Model file for the job. Use its own axes, mm. Face numbers are marked on the shaded views. A direction names the side the tool comes from. Coordinates: 2 decimals unless noted, no trailing zeros. Write each loop counter-clockwise with the first axis right and the second up, starting at its lowest first coordinate (ties: lowest second). Pieces come first, ordered by that corner, then holes. Notation, with made-up numbers: M 73.5,85 L 88.5,85 A14 cw 88.5,91 Z; hole C 3.5,-4 d2. An arc over 180 degrees is marked long. Answer in a Markdown table with one row per item. Add a question column.
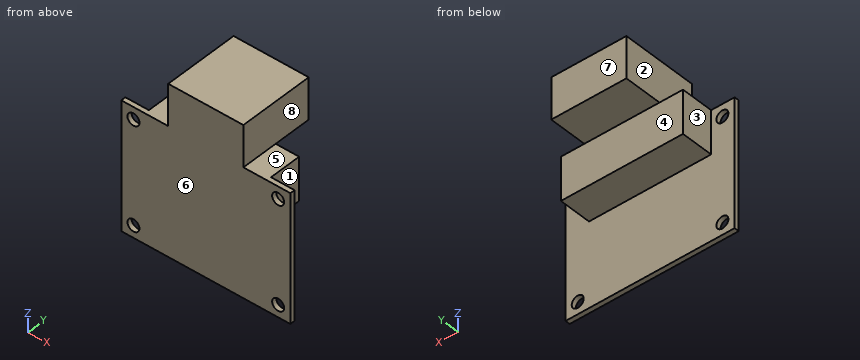
```python
from build123d import *

# Parameters (mm, degrees)
SKETCH1_W            = 45
SKETCH1_H            = 45
BOSS_EXTRUDE1_DEPTH  = 10.033
SKETCH2_W            = 12.5
SKETCH2_H            = 11
CUT_EXTRUDE1_DEPTH   = 20.066
CUT_EXTRUDE2_DEPTH   = 18.796
CUT_EXTRUDE3_DEPTH   = 10.16
M3_CLEARANCE_HOLE1_D = 3.2


with BuildPart() as part:
    # Sketch1 → Boss-Extrude1 (new, symmetric)
    with BuildSketch(Plane(origin=(0, 0, 0), x_dir=(1, 0, 0), z_dir=(0, 1, 0))):
        Rectangle(SKETCH1_W, SKETCH1_H)
    extrude(amount=BOSS_EXTRUDE1_DEPTH, both=True)

    # Sketch2 → Cut-Extrude1 (cut)
    with BuildSketch(Plane(origin=(0, 10.033, 0), x_dir=(1, 0, 0), z_dir=(0, 1, 0))):
        with Locations((16.25, -17)):
            Rectangle(SKETCH2_W, SKETCH2_H)
    cut_extrude1 = extrude(amount=-CUT_EXTRUDE1_DEPTH, mode=Mode.SUBTRACT)

    # Mirror1: Cut-Extrude1 across plane
    add(cut_extrude1.mirror(Plane(origin=(0, 0, 0), x_dir=(0, 0, 1), z_dir=(1, 0, 0))), mode=Mode.SUBTRACT)

    # Sketch3 → Cut-Extrude2 (cut)
    with BuildSketch(Plane(origin=(0, 10.033, 0), x_dir=(1, 0, 0), z_dir=(0, 1, 0))):
        Polygon((-22.5, -11.5), (-16.25, -11.5), (-16.25, 0), (16.248560403, 0), (16.248560403, -11.5), (22.5, -11.5), (22.5, 22.5), (-22.5, 22.5), align=None)
    extrude(amount=-CUT_EXTRUDE2_DEPTH, mode=Mode.SUBTRACT)

    # Sketch3<3> → Cut-Extrude3 (cut)
    with BuildSketch(Plane(origin=(0, 10.033, 0), x_dir=(1, 0, 0), z_dir=(0, 1, 0))):
        Polygon((-16.25, 0), (-16.25, -11.5), (-10, -11.5), (10, -11.5), (16.248560403, -11.5), (16.248560403, 0), align=None)
    extrude(amount=-CUT_EXTRUDE3_DEPTH, mode=Mode.SUBTRACT)

    # M3 Clearance Hole1 (through all)
    with Locations(Plane(origin=(0, -8.763, 0), x_dir=(1, 0, 0), z_dir=(0, 1, 0))):
        with Locations((-19.25, 19.25), (-19.25, -8.25), (19.25, -8.25), (19.25, 19.25)):
            Hole(M3_CLEARANCE_HOLE1_D / 2)


solid = part.part
```
1) Slice it at D-D (x = 2). Give the cut face in (y, z), then the cut area to 3 significant figures.
2) Flat gauge pins, fed straight in: pin 1 Ø9 at (y, z) = (3, 17.5) entering from -X; pin 2 Ø3 at (y, z) = (-3.5, 2.5) entering from +X; pin 3 Ø5 at (x, y) = (4, 6) entering from -Z; pin 4 Ø4 at (x, z) = (19.25, -19.25) entering from -Y. Where does each tip first touch, or does it go through?
3) Drill centre lines: probe 1 along Z at (x, y) = (-19.25, -9.25); probe 2 along X at (y, z) = (-9.35, 8.25); probe 3 along Y at (x, z) = (18, -15.5). Where is each one in solid material? Low to high.
4) Slice it at C-C (y = -6.5). Give the cut face in (x, z).
5) Which spindle directions (+Z, -Z, +X, -X, +Y, -Y) get a long thin tool onto all of the face, cutting with end or side? Do the marked faces 1, 2, 3, 4 and 5. Say none if no direction does.
6) Slice it at A-A (x = -19.25). Give the cut face in (y, z), then the cut area to 3 significant figures.
7) Slice it at B-B (z = 8.25). Give the cut face in (x, y), then the cut area to 3 significant figures.
8) Two-plate mould, pull along Y, no slides. Class the marked faces 6, 7 and 8: released by +Y, released by -Y, zero draft, split by the parting line, or undercut.
Ans:
| question | item | result |
|---|---|---|
| 1 | outline | M -10.03,-22.5 L -8.76,-22.5 L -8.76,0 L -0.13,0 L -0.13,11.5 L 10.03,11.5 L 10.03,22.5 L -10.03,22.5 Z |
| 1 | area | 363 mm2 |
| 2 | pin 1 | stops at x = -10 |
| 2 | pin 2 | stops at x = 16.25 |
| 2 | pin 3 | stops at z = 11.5 |
| 2 | pin 4 | stops at y = -10.03 |
| 3 | probe 1 | z = -22.5 to -20.85, -17.65 to 6.65, 9.85 to 11.5 |
| 3 | probe 2 | x = -22.5 to -20.85, -17.65 to 17.65, 20.85 to 22.5 |
| 3 | probe 3 | y = -10.03 to -8.76 |
| 4 | outline | M -16.25,0 L 16.25,0 L 16.25,11.5 L 10,11.5 L 10,22.5 L -10,22.5 L -10,11.5 L -16.25,11.5 Z |
| 5 | face 1 | +Z, -Z, +X, +Y |
| 5 | face 2 | +Z, -X, +Y, -Y |
| 5 | face 3 | +Z, -Z, -X, +Y |
| 5 | face 4 | -Z, +X, -X, +Y |
| 5 | face 5 | +Z, +X, +Y, -Y |
| 6 | outline | M -10.03,-22.5 L -8.76,-22.5 L -8.76,-20.85 L -10.03,-20.85 Z; M -10.03,-17.65 L -8.76,-17.65 L -8.76,6.65 L -10.03,6.65 Z; M -10.03,9.85 L -8.76,9.85 L -8.76,11.5 L -10.03,11.5 Z |
| 6 | area | 35.1 mm2 |
| 7 | outline | M -22.5,-10.03 L -20.85,-10.03 L -20.85,-8.76 L -22.5,-8.76 Z; M -17.65,-10.03 L 17.65,-10.03 L 17.65,-8.76 L 16.25,-8.76 L 16.25,-0.13 L -16.25,-0.13 L -16.25,-8.76 L -17.65,-8.76 Z; M 20.85,-10.03 L 22.5,-10.03 L 22.5,-8.76 L 20.85,-8.76 Z |
| 7 | area | 330 mm2 |
| 8 | face 6 | released by -Y |
| 8 | face 7 | released by +Y |
| 8 | face 8 | zero draft |
